Check sheet for the modelled part. Datum: model origin and axes. Units: mm. Give positions to 0.01 mm unless a question says otherwise; leave off trailing zeros. Write each loop counter-clockwise with the first axis right and the second up, starting at its lowest first coordinate (ties: lowest second). Pieces come first, ordered by that corner, then holes. Notation, with made-up numbers: (85.5, 42.25) -> (134.5, 42.25) arc R14 ccw to (134.5, 48.25) -> close; hole circle Ø11 at (-1.75, 73.25). An arc over 180 degrees is marked (long way). Use a Markdown table: item, result. Add a question column.
1. Scan lines: probe 1 along X at (y, z) = (6.25, 1.2); probe 2 along Y at (x, z) = (-10.5, 0.85); probe 3 along X at (y, z) = (-6.25, 1). Record each from-to range of solid material in increasing order. Write a range as [from, to].
2. Cross-section at B-B (x = 15). Enter the section's corners in (y, z).
3. Cross-section at A-A (y = -3.25). Enter the section's corners in (x, z).
4. Gauge pin test, flat ends, axial feed: P1, Ø0.9, axis at x = -9, y = -7.5, coming from the -Z side; P2, Ø5, axis at x = 3, y = 3, coming from the -Z side; P3, Ø3, axis at y = 5.5, z = 1, coming from the +X side; P4, Ø1.3, axis at x = -10.5, y = -6.25, coming from the -Z side. Record the tip position at first contact, or that the pin passes through.
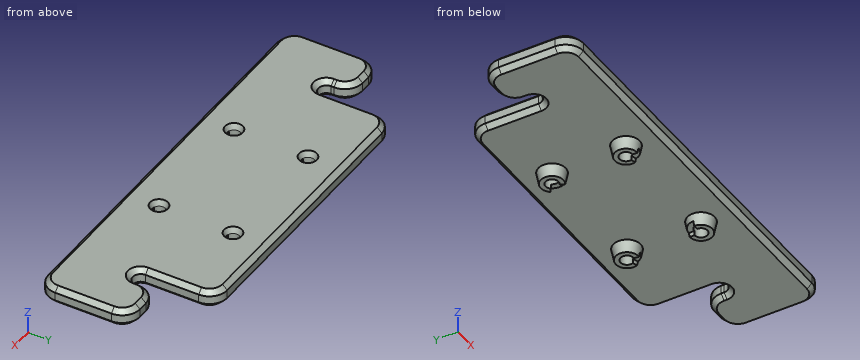
from build123d import *
from OCP.BRepFilletAPI import BRepFilletAPI_MakeChamfer

# Parameters (mm, degrees)
BOSS_EXTRUDE1_DEPTH            = 3
SKETCH4_R                      = 2.3
BOSS_EXTRUDE2_DEPTH            = 2
M2_CLEARANCE_HOLE1_D           = 2.2
M2_CLEARANCE_HOLE1_CSINK_D     = 3
M2_CLEARANCE_HOLE1_CSINK_ANGLE = 45
BOSS_EXTRUDE3_START            = -1
BOSS_EXTRUDE3_DEPTH            = 0.75
CHAMFER1_SIZE                  = 0.4
CHAMFER1_SIZE_2                = 2
CUT_EXTRUDE2_START             = -0.8
CUT_EXTRUDE2_DEPTH             = 0.8
CUT_EXTRUDE3_DEPTH             = 38.336309405
FILLET1_R                      = 3
CHAMFER2_SIZE                  = 0.8


with BuildPart() as part:
    # Sketch1 → Boss-Extrude1 (new body)
    with BuildSketch(Plane.XY):
        with BuildLine():
            Line((32, 12), (-32, 12))
            ThreePointArc((-32, 12), (-34.121320344, 11.121320344), (-35, 9))
            Line((-35, 9), (-35, -9))
            ThreePointArc((-35, -9), (-34.121320344, -11.121320344), (-32, -12))
            Line((-32, -12), (32, -12))
            ThreePointArc((32, -12), (34.121320344, -11.121320344), (35, -9))
            Line((35, -9), (35, 9))
            ThreePointArc((35, 9), (34.121320344, 11.121320344), (32, 12))
        make_face()
    extrude(amount=BOSS_EXTRUDE1_DEPTH)

    # Sketch4 → Boss-Extrude2 (add)
    with BuildSketch(Plane(origin=(0, 0, 0), x_dir=(-1, 0, 0), z_dir=(0, 0, -1))):
        with Locations((-10.5, 6.25)):
            Circle(SKETCH4_R)
        with Locations((10.5, 6.25)):
            Circle(SKETCH4_R)
        with Locations((10.5, -6.25)):
            Circle(SKETCH4_R)
        with Locations((-10.5, -6.25)):
            Circle(SKETCH4_R)
    extrude(amount=BOSS_EXTRUDE2_DEPTH)

    # M2 Clearance Hole1 (through all)
    with Locations(Plane.XY.offset(3)):
        with Locations((10.5, 6.25), (10.5, -6.25), (-10.5, -6.25), (-10.5, 6.25)):
            CounterSinkHole(M2_CLEARANCE_HOLE1_D / 2, M2_CLEARANCE_HOLE1_CSINK_D / 2, counter_sink_angle=M2_CLEARANCE_HOLE1_CSINK_ANGLE)

    # Sketch6 → Boss-Extrude3 (add)
    with BuildSketch(Plane.XY.offset(3).offset(BOSS_EXTRUDE3_START)):
        with BuildLine():
            Line((10.124367201, 5.15), (10.875632799, 5.15))
            ThreePointArc((10.875632799, 5.15), (10.5, 5.32), (10.124367201, 5.15))
        make_face()
        with BuildLine():
            Line((10.124367201, 7.35), (10.875632799, 7.35))
            ThreePointArc((10.875632799, 7.35), (10.5, 7.18), (10.124367201, 7.35))
        make_face()
        with BuildLine():
            Line((-10.124367201, 5.15), (-10.875632799, 5.15))
            ThreePointArc((-10.875632799, 5.15), (-10.5, 5.32), (-10.124367201, 5.15))
        make_face()
        with BuildLine():
            Line((-10.124367201, 7.35), (-10.875632799, 7.35))
            ThreePointArc((-10.875632799, 7.35), (-10.5, 7.18), (-10.124367201, 7.35))
        make_face()
        with BuildLine():
            Line((10.124367201, -7.35), (10.875632799, -7.35))
            ThreePointArc((10.875632799, -7.35), (10.5, -7.18), (10.124367201, -7.35))
        make_face()
        with BuildLine():
            Line((10.124367201, -5.15), (10.875632799, -5.15))
            ThreePointArc((10.875632799, -5.15), (10.5, -5.32), (10.124367201, -5.15))
        make_face()
        with BuildLine():
            Line((-10.124367201, -7.35), (-10.875632799, -7.35))
            ThreePointArc((-10.875632799, -7.35), (-10.5, -7.18), (-10.124367201, -7.35))
        make_face()
        with BuildLine():
            Line((-10.124367201, -5.15), (-10.875632799, -5.15))
            ThreePointArc((-10.875632799, -5.15), (-10.5, -5.32), (-10.124367201, -5.15))
        make_face()
    extrude(amount=-BOSS_EXTRUDE3_DEPTH)

    # Chamfer1
    chamfer1_edges_1 = [part.edges().sort_by_distance(p)[0] for p in [
        (12.8, 6.25, -2),
    ]]
    chamfer1_side_1 = [part.faces().sort_by_distance(p)[0] for p in [
        (12.792, 6.25, -2),
    ]]
    chamfer1_edges_2 = [part.edges().sort_by_distance(p)[0] for p in [
        (-8.2, 6.25, -2),
    ]]
    chamfer1_side_2 = [part.faces().sort_by_distance(p)[0] for p in [
        (-8.208, 6.25, -2),
    ]]
    chamfer1_edges_3 = [part.edges().sort_by_distance(p)[0] for p in [
        (-8.2, -6.25, -2),
    ]]
    chamfer1_side_3 = [part.faces().sort_by_distance(p)[0] for p in [
        (-8.208, -6.25, -2),
    ]]
    chamfer1_edges_4 = [part.edges().sort_by_distance(p)[0] for p in [
        (12.8, -6.25, -2),
    ]]
    chamfer1_side_4 = [part.faces().sort_by_distance(p)[0] for p in [
        (12.792, -6.25, -2),
    ]]
    chamfer1 = BRepFilletAPI_MakeChamfer(part.part.solid().wrapped)
    for e in chamfer1_edges_1:
        chamfer1.Add(CHAMFER1_SIZE - 0.0001, CHAMFER1_SIZE_2 - 0.0001, e.wrapped, chamfer1_side_1[0].wrapped)
    for e in chamfer1_edges_2:
        chamfer1.Add(CHAMFER1_SIZE - 0.0001, CHAMFER1_SIZE_2 - 0.0001, e.wrapped, chamfer1_side_2[0].wrapped)
    for e in chamfer1_edges_3:
        chamfer1.Add(CHAMFER1_SIZE - 0.0001, CHAMFER1_SIZE_2 - 0.0001, e.wrapped, chamfer1_side_3[0].wrapped)
    for e in chamfer1_edges_4:
        chamfer1.Add(CHAMFER1_SIZE - 0.0001, CHAMFER1_SIZE_2 - 0.0001, e.wrapped, chamfer1_side_4[0].wrapped)
    add(Compound.cast(chamfer1.Shape()), mode=Mode.REPLACE)  # a hair under: the kernel refuses the full size

    # Sketch5 → Cut-Extrude2 (cut)
    with BuildSketch(Plane(origin=(0, 0, -2), x_dir=(-1, 0, 0), z_dir=(0, 0, -1)).offset(CUT_EXTRUDE2_START)):
        with BuildLine():
            Line((8.712564289, 7.697436899), (10.5, 6.25))
            Line((10.5, 6.25), (9.180774196, 4.365950298))
            ThreePointArc((9.180774196, 4.365950298), (8.222383442, 5.929901868), (8.712564289, 7.697436899))
        make_face()
        with BuildLine():
            Line((10.419731158, -8.548598902), (10.5, -6.25))
            Line((10.5, -6.25), (8.258948851, -6.767387425))
            ThreePointArc((8.258948851, -6.767387425), (9.037020093, -8.024736542), (10.419731158, -8.548598902))
        make_face()
        with BuildLine():
            Line((-12.674692724, 5.501193245), (-10.5, 6.25))
            Line((-10.5, 6.25), (-10.740415466, 3.962599641))
            ThreePointArc((-10.740415466, 3.962599641), (-11.931783664, 4.450001239), (-12.674692724, 5.501193245))
        make_face()
        with BuildLine():
            Line((-10.5, -3.95), (-10.5, -6.25))
            Line((-10.5, -6.25), (-8.200350301, -6.209859465))
            ThreePointArc((-8.200350301, -6.209859465), (-8.887908692, -4.609523967), (-10.5, -3.95))
        make_face()
    extrude(amount=CUT_EXTRUDE2_DEPTH, mode=Mode.SUBTRACT)

    # Sketch7 → Cut-Extrude3 (cut, through all)
    with BuildSketch(Plane.XY.offset(3)):
        with BuildLine():
            Line((35, 3.5), (27.35, 3.5))
            Line((27.35, 3.5), (27.35, 0))
            ThreePointArc((27.35, 0), (26, -1.35), (24.65, 0))
            Line((24.65, 0), (24.65, 12))
            Line((24.65, 12), (35, 12))
            Line((35, 12), (35, 3.5))
        make_face()
        with BuildLine():
            Line((-35, 12), (-24.65, 12))
            Line((-24.65, 12), (-24.65, 0))
            ThreePointArc((-24.65, 0), (-26, -1.35), (-27.35, 0))
            Line((-27.35, 0), (-27.35, 3.5))
            Line((-27.35, 3.5), (-35, 3.5))
            Line((-35, 3.5), (-35, 12))
        make_face()
    extrude(amount=-CUT_EXTRUDE3_DEPTH, mode=Mode.SUBTRACT)

    # Fillet1
    fillet1_edges = [part.edges().sort_by_distance(p)[0] for p in [
        (24.65, 12, 1.5),
        (35, 3.5, 1.5),
        (27.35, 3.5, 1.5),
        (-35, 3.5, 1.5),
        (-27.35, 3.5, 1.5),
        (-24.65, 12, 1.5),
    ]]
    fillet(fillet1_edges, radius=FILLET1_R)

    # Chamfer2
    chamfer2_edges = [part.edges().sort_by_distance(p)[0] for p in [
        (35, -4.25, 0),
        (34.121320344, -11.121320344, 0),
        (0, -12, 0),
        (-34.121320344, -11.121320344, 0),
        (34.121320344, -11.121320344, 3),
        (35, -4.25, 3),
        (-26, -1.35, 0),
        (-27.35, 0.25, 0),
        (24.65, 4.5, 0),
        (26, -1.35, 0),
        (26, -1.35, 3),
        (27.35, 0.25, 3),
        (-26, -1.35, 3),
        (-24.65, 4.5, 3),
        (-31.175, 3.5, 0),
        (-31.175, 3.5, 3),
        (31.175, 3.5, 3),
        (24.65, 4.5, 3),
        (0, 12, 3),
        (-27.35, 0.25, 3),
        (-35, -4.25, 3),
        (34.121320344, 2.621320344, 3),
        (28.228679656, 2.621320344, 3),
        (23.771320344, 11.121320344, 3),
        (-23.771320344, 11.121320344, 3),
        (-28.228679656, 2.621320344, 3),
        (-34.121320344, 2.621320344, 3),
        (-35, -4.25, 0),
        (31.175, 3.5, 0),
        (-24.65, 4.5, 0),
        (0, 12, 0),
        (27.35, 0.25, 0),
        (34.121320344, 2.621320344, 0),
        (28.228679656, 2.621320344, 0),
        (23.771320344, 11.121320344, 0),
        (-23.771320344, 11.121320344, 0),
        (-28.228679656, 2.621320344, 0),
        (-34.121320344, 2.621320344, 0),
        (-34.121320344, -11.121320344, 3),
        (0, -12, 3),
    ]]
    chamfer(chamfer2_edges, length=CHAMFER2_SIZE)


solid = part.part
Worked answers:
| question | item | result |
|---|---|---|
| 1 | probe 1 | x = [-24.65, -11.6], [-9.4, 9.4], [11.6, 24.65] |
| 1 | probe 2 | y = [-12, -7.35], [-5.15, 5.15], [7.35, 12] |
| 1 | probe 3 | x = [-35, -11.6], [-9.4, 9.4], [11.6, 35] |
| 2 | outline | (-12, 0.8) -> (-11.2, 0) -> (11.2, 0) -> (12, 0.8) -> (12, 2.2) -> (11.2, 3) -> (-11.2, 3) -> (-12, 2.2) -> close |
| 3 | outline | (-35, 0.8) -> (-34.2, 0) -> (34.2, 0) -> (35, 0.8) -> (35, 2.2) -> (34.2, 3) -> (-34.2, 3) -> (-35, 2.2) -> close |
| 4 | P1 | stops at z = -1.2 |
| 4 | P2 | stops at z = 0 |
| 4 | P3 | stops at x = 24.65 |
| 4 | P4 | passes through |
